Here's how the part is built. I have some questions about the finished solid (model axes, mm). Give positions to 0.01 mm unless a question says otherwise; leave off trailing zeros. Write each loop counter-clockwise with the first axis right and the second up, starting at its lowest first coordinate (ties: lowest second). Pieces come first, ordered by that corner, then holes. Notation, with made-up numbers: (88.5, 20) -> (109.5, 20) arc R22 cw to (109.5, 59) -> close; hole circle Ø2 at (18, -1). An arc over 180 degrees is marked (long way). Use CSV: the item, a comma, the result in double quotes. Start each with the question number.
(1) Suppose I cut it at A-A on z = -110.5. List the corners of the cut face in (x, y) for me.
(2) I need wall thicknesses on L1, parallel to Z at x = 31, y = -0.7; L2, parallel to X at y = -1.3, z = -77; L3, parallel to X at y = -0.8, z = -101.5. Which ranges of each line are inside material? Lowest first, please. Write a range as [from, to].
(3) Suppose I cut it at D-D on z = -80. List the corners of the cut face in (x, y) for me, plus the area to 3 significant figures.
(4) Suppose I cut it at C-C on x = -49.5. List the corners of the cut face in (y, z) for me.
(5) For pin 1 Ø1.5 at (x, z) = (88.5, -50) entering from +Y, with a flat end and sliding along its axis, tell me the tip position at first contact or that it passes through.
(6) Suppose I cut it at B-B on y = -2.5. List the corners of the cut face in (x, z) for me.
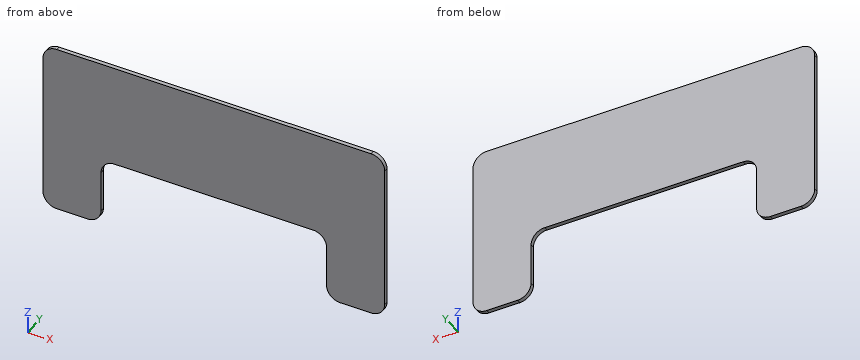
from build123d import *

# Parameters (mm, degrees)
BASE_FLANGE1_DEPTH = 3


# Sheet-metal steps are written as plain solids
with BuildPart() as part:
    # Sketch16 → Base-Flange1 (new body)
    with BuildSketch(Plane(origin=(0, 0, 0), x_dir=(1, 0, 0), z_dir=(0, 1, 0))):
        with BuildLine():
            Line((-50, 0), (50, 0))
            Line((50, 0), (115, 0))
            ThreePointArc((115, 0), (122.071067812, 2.928932188), (125, 10))
            Line((125, 10), (125, 75))
            Line((125, 75), (125, 115))
            ThreePointArc((125, 115), (122.071067812, 122.071067812), (115, 125))
            Line((115, 125), (92.5, 125))
            ThreePointArc((92.5, 125), (85.428932188, 122.071067812), (82.5, 115))
            Line((82.5, 115), (82.5, 85))
            ThreePointArc((82.5, 85), (79.571067812, 77.928932188), (72.5, 75))
            Line((72.5, 75), (50, 75))
            Line((50, 75), (-50, 75))
            Line((-50, 75), (-72.5, 75))
            ThreePointArc((-72.5, 75), (-79.571067812, 77.928932188), (-82.5, 85))
            Line((-82.5, 85), (-82.5, 115))
            ThreePointArc((-82.5, 115), (-85.428932188, 122.071067812), (-92.5, 125))
            Line((-92.5, 125), (-115, 125))
            ThreePointArc((-115, 125), (-122.071067812, 122.071067812), (-125, 115))
            Line((-125, 115), (-125, 75))
            Line((-125, 75), (-125, 10))
            ThreePointArc((-125, 10), (-122.071067812, 2.928932188), (-115, 0))
            Line((-115, 0), (-50, 0))
        make_face()
    extrude(amount=-BASE_FLANGE1_DEPTH)


solid = part.part
Geometry says:
1,outline,"(-125, -3) -> (-82.5, -3) -> (-82.5, 0) -> (-125, 0) -> close; (82.5, -3) -> (125, -3) -> (125, 0) -> (82.5, 0) -> close"
2,L1,"[-75, 0]"
2,L2,"[-125, -78.5], [78.5, 125]"
2,L3,"[-125, -82.5], [82.5, 125]"
3,outline,"(-125, -3) -> (-81.16, -3) -> (-81.16, 0) -> (-125, 0) -> close; (81.16, -3) -> (125, -3) -> (125, 0) -> (81.16, 0) -> close"
3,area,"263 mm²"
4,outline,"(-3, -75) -> (0, -75) -> (0, 0) -> (-3, 0) -> close"
5,pin 1,"y = 0"
6,outline,"(-125, -115) arc R10 ccw to (-115, -125) -> (-92.5, -125) arc R10 ccw to (-82.5, -115) -> (-82.5, -85) arc R10 cw to (-72.5, -75) -> (72.5, -75) arc R10 cw to (82.5, -85) -> (82.5, -115) arc R10 ccw to (92.5, -125) -> (115, -125) arc R10 ccw to (125, -115) -> (125, -10) arc R10 ccw to (115, 0) -> (-115, 0) arc R10 ccw to (-125, -10) -> close"
